```python
from build123d import *

# Parameters (mm, degrees)
F0_W     = 482.6
F0_H     = 177.8
F1_DEPTH = 477.52
F4_DEPTH = 9.525
F5_R     = 4.445


# Not quite as in the source:
# - a pattern or mirror of a feature is missing from the dataset's text; its kind, count and spacing are read off the source's solid


with BuildPart() as f1:
    # F0 (on Front) → F1 (new body)
    with BuildSketch(Plane.XZ):
        Rectangle(F0_W, F0_H)
    extrude(amount=-F1_DEPTH)

    # F3 (on offset) → F4 (join)
    with BuildSketch(Plane.YZ.offset(241.3)):
        Polygon((0, 73.025), (0, 82.55), (-45.2747344971, 82.55), (-45.2747344971, -82.55), (0, -82.55), (0, -73.025), (-35.7497344971, -73.025), (-35.7497344971, 73.025), align=None)
    f4 = extrude(amount=-F4_DEPTH)

    # F4_copies: F4 across plane
    add(f4.mirror(Plane(origin=(0, 0, 0), x_dir=(0, 0, -1), z_dir=(-1, 0, 0))))

    # F5
    f5_edges = [f1.edges().sort_by_distance(p)[0] for p in [
        (236.5375, -45.274734, 82.55),
        (236.5375, -45.274734, -82.55),
        (236.5375, -35.749734, -73.025),
        (236.5375, -35.749734, 73.025),
        (-236.5375, -45.274734, -82.55),
        (-236.5375, -35.749734, -73.025),
        (-236.5375, -35.749734, 73.025),
        (-236.5375, -45.274734, 82.55),
    ]]
    fillet(f5_edges, radius=F5_R)


solid = f1.part
```
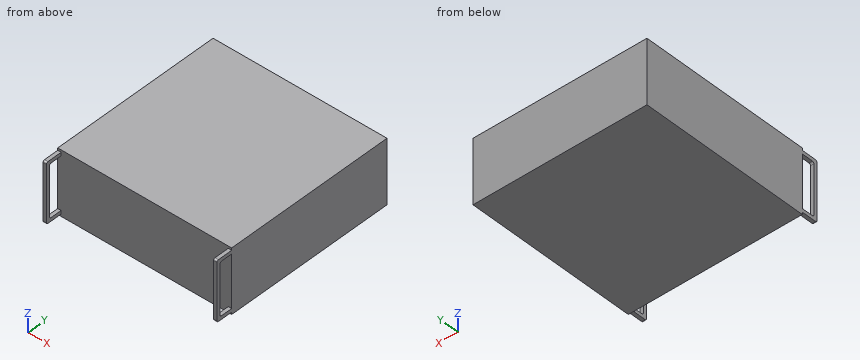
Design review of the part built by this model. Coordinates are the model's own, in mm. Coordinates: 2 decimals unless noted, no trailing zeros. Order: outer loops, then holes, each group sorted by start corner. A loop starts at its lowest first (then second) coordinate and runs counter-clockwise, first axis right, second up. Notation, with made-up numbers: M 46,72.25 L 72,72.25 A19 cw 72,84.25 Z; hole C 36.5,88 d7. An arc over 180 degrees is marked long. Answer as a JSON object with one key per item and string values. Group by question number.
1) Wall thickness on L1, parallel to Y at x = -153.5, z = 65.5: over which ranges is the line inside the solid? List them lowest first.
2) Add section B-B, the plane x = 207.5. Write out the cut boundary in (y, z), then the cut area to 3 significant figures.
3) For pin 1 (10.5 mm diameter, centred on x = 237, y = -9, fed in from -Z); pin 2 (10.5 mm diameter, centred on x = 237.5, y = -22.5, fed in from +Z); pin 3 (7.5 mm diameter, centred on x = -238, y = -11.5, fed in from +Z), all flat-tipped, find the tip position at first contact; note any pin that passes through.
4) Add section A-A, the plane z = -36. Write out the cut boundary in (x, y) (3 decimals).
Computed values:
{
 "1": {"L1": "y = 0 to 477.52"},
 "2": {"outline": "M 0,-88.9 L 477.52,-88.9 L 477.52,88.9 L 0,88.9 Z", "area": "84,900 mm^2"},
 "3": {"pin 1": "stops at z = -82.55", "pin 2": "stops at z = 82.55", "pin 3": "stops at z = 82.55"},
 "4": {"outline": "M -241.3,-45.275 L -231.775,-45.275 L -231.775,-35.75 L -241.3,-35.75 Z; M -241.3,0 L 241.3,0 L 241.3,477.52 L -241.3,477.52 Z; M 231.775,-45.275 L 241.3,-45.275 L 241.3,-35.75 L 231.775,-35.75 Z"}
}
